Part model, mm, in its own coordinate system. A direction names the side the tool comes from. Give positions to 0.01 mm unless a question says otherwise; leave off trailing zeros. Loops run counter-clockwise (first coordinate to the right, second up) from the corner with the lowest first, then second, coordinate; pieces in that order, holes last. Notation, with made-up numbers: M -24,0.25 L -7,0.25 A32 ccw -7,34.25 Z; hole C 20.5,55.25 d11. An arc over 180 degrees is marked long. Put each result on its own line as item: value. Start each with the question number.
```python
from build123d import *

# Parameters (mm, degrees)
SKETCH_1_W          = 12
SKETCH_1_H          = 4
SKETCH_1_R          = 1.5
EXTRUDE_1_DEPTH     = 6
SKETCH_2_R          = 1.5
EXTRUDE_2_DEPTH     = 3
CUT_EXTRUDE_1_REACH = 15.118
SKETCH_3_R          = 1.4


with BuildPart() as part:
    # Эскиз1 → Бобышка-Вытянуть1 (new body)
    with BuildSketch(Plane.XY):
        with Locations((4.958157727, 0.498048464)):
            Rectangle(SKETCH_1_W, SKETCH_1_H)
        with Locations((8.958157727, 0.498048464)):
            Circle(SKETCH_1_R, mode=Mode.SUBTRACT)
    extrude(amount=EXTRUDE_1_DEPTH)

    # Эскиз2 → Бобышка-Вытянуть2 (add)
    with BuildSketch(Plane(origin=(0, 0, 0), x_dir=(-1, 0, 0), z_dir=(0, 0, -1))):
        with Locations(Location((-0.958157727, 0.498048464, 0), (0, 0, 180))):
            Circle(SKETCH_2_R)
    extrude(amount=EXTRUDE_2_DEPTH)

    # Эскиз3 → Вырез-Вытянуть1 (cut, up to next)
    with BuildSketch(Plane.XZ.offset(1.501951536), mode=Mode.PRIVATE) as cut_extrude_1_sk1:
        with Locations((4.958157727, 3)):
            Circle(SKETCH_3_R)
    cut_extrude_1_tool1 = extrude(cut_extrude_1_sk1.sketch, amount=-CUT_EXTRUDE_1_REACH, mode=Mode.PRIVATE) & part.part
    add(cut_extrude_1_tool1.solids().sort_by_distance((4.958158, -1.501952, 3))[0], mode=Mode.SUBTRACT)


solid = part.part
```
1) Band-saw the part on D-D on y = -0.45. Give the cut face in (x, z), then the cut area to 3 significant figures.
2) Which spindle directions (+Z, -Z, +X, -X, +Y, -Y) get a long thin tool onto all of the face, cutting with end or side? Do faces 1 (the cylindrical face through (0.63, 1.96, -1.48)), 2 (the flat face through (3.5, -1.502, 2.3)). Say none if no direction does.
3) Wall check: L1, parallel to X at y = -0.7, z = 3.25; L2, parallel to Z at x = 9.5, y = -1.3; L3, parallel to Z at x = 4.5, y = 2.25. Give the ranges that are in metal, low to high.
4) Band-saw the part on C-C on x = 4.25. Give the cut face in (y, z).
5) Pin check, flat tip, straight feed: pin 1 Ø2 at (x, z) = (4.96, 3) entering from +Y. Stop position of the tip, or through.
6) Mould opens along X. For faces 3 (the flat face through (4, 1, 6)), 4 (the flat face through (-1.042, 0, 3)), 5 (the cylindrical face through (10.344, -0.076, 2.958)), 6 (the cylindrical face through (3.847, 0.47, 2.148)) say: +X half, -X half, draft (parallel to the pull), parting line (faces both ways), or undercut.
7) Band-saw the part on A-A on y = 0.25. Give the cut face in (x, z).
8) Band-saw the part on B-B on z = 3. Give the cut face in (x, y).
Evaluation:
1. outline: M -1.04,0 L -0.2,0 L -0.2,-3 L 2.12,-3 L 2.12,0 L 7.8,0 L 7.8,6 L -1.04,6 Z; M 10.12,0 L 10.96,0 L 10.96,6 L 10.12,6 Z; hole C 4.96,3 d2.8
1. area: 58.9 mm2
2. face 1: -Z
2. face 2: +Z, -Z, +X, -X, -Y
3. L1: -1.04 to 3.58, 6.34 to 8.06, 9.86 to 10.96
3. L2: 0 to 6
3. L3: 0 to 1.68, 4.32 to 6
4. outline: M -1.5,0 L 2.5,0 L 2.5,1.79 L -1.5,1.79 Z; M -1.5,4.21 L 2.5,4.21 L 2.5,6 L -1.5,6 Z
5. pin 1: through
6. face 3: draft
6. face 4: -X half
6. face 5: undercut
6. face 6: undercut
7. outline: M -1.04,0 L -0.52,0 L -0.52,-3 L 2.44,-3 L 2.44,0 L 7.48,0 L 7.48,6 L -1.04,6 Z; M 10.44,0 L 10.96,0 L 10.96,6 L 10.44,6 Z; hole C 4.96,3 d2.8
8. outline: M -1.04,-1.5 L 3.56,-1.5 L 3.56,2.5 L -1.04,2.5 Z; M 6.36,-1.5 L 10.96,-1.5 L 10.96,2.5 L 6.36,2.5 Z; hole C 8.96,0.5 d3
